CAD build for the part. Positions are in the model's coordinates, mm. Coordinates: 2 decimals unless noted, no trailing zeros. Order: outer loops, then holes, each group sorted by start corner. A loop starts at its lowest first (then second) coordinate and runs counter-clockwise, first axis right, second up. Notation, with made-up numbers: (69, 88) - (128, 88) arc R18 ccw to (128, 100) - close; hole circle Ø9 at (4, 14.25). An arc over 180 degrees is marked (long way). Write each question's results on one line, items separated by ' | '. Start each with the question number.
Q1. Band-saw the part on B-B, the plane x = 27.5. Write the cut outline in (y, z).
Q2. Band-saw the part on D-D, the plane x = -60.5. Write the cut outline in (y, z), then the cut area to 3 significant figures.
Q3. Band-saw the part on A-A, the plane z = 2. Count the separate pieces of the cut face and the enclosed holes in it, then the cut area to 3 significant figures.
Q4. Pin check, flat tip, straight feed: P1, Ø1.5, axis at y = 52, z = 0.5, coming from the +X side. Stop position of the tip, or through.
Q5. Band-saw the part on C-C, the plane y = 20.5. Write the cut outline in (x, z).
Q6. Wall check: probe 1 along Y at (x, z) = (60.5, 1.6); probe 2 along Y at (x, z) = (27.5, 1.4); probe 3 along X at (y, z) = (-56, 0.6). Give the ranges that are in metal, low to high.
Autodesk Inventor part; units mm, degrees
ref_plane "YZ Plane" through (0, 0, 0) normal (1, 0, 0) x (0, 1, 0)
ref_plane "XZ Plane" through (0, 0, 0) normal (0, 1, 0) x (-1, 0, 0)
ref_plane "XY Plane" through (0, 0, 0) normal (0, 0, 1) x (1, 0, 0)
sketch "Sketch1" plane through (0, 0, 0) normal (0, 0, 1) x (1, 0, 0)
  line L0 (-72.5, 65) -> (72.5, 65)
  line L1 (72.5, 65) -> (72.5, -65)
  line L2 (72.5, -65) -> (-72.5, -65)
  line L3 (-72.5, -65) -> (-72.5, 65)
  point P0 (0, 0)
  dimension "d0" = 145
  dimension "d1" = 130
  dimension "d2" = 65
  dimension "d3" = 72.5
extrude "profile" add sketch "Sketch1" along normal blind 2.6568
sketch "Sketch2" plane through (0, 0, 2.6568) normal (0, 0, 1) x (1, 0, 0)
  line L0 (72.5, 65) -> (-72.5, 65)
  line L1 (-72.5, 65) -> (-72.5, -65)
  line L2 (-32.5, 35) -> (-7.5, 35) construction
  line L3 (-32.5, 32.25) -> (-7.5, 32.25)
  line L4 (-7.5, 37.75) -> (-32.5, 37.75)
  arc A0 (-32.5, 37.75) -> (-32.5, 32.25) centre (-32.5, 35) ccw
  arc A1 (-7.5, 32.25) -> (-7.5, 37.75) centre (-7.5, 35) ccw
  point P0 (0, 0)
  point P1 (-20, 35)
  dimension "d6" = 25
  dimension "d7" = 5.5
  dimension "d8" = 30
  dimension "d9" = 40
extrude "x_slots" cut sketch "Sketch2" against normal through all
pattern_linear "Rectangular Pattern1" count 2 spacing 20 along (0, -1, 0) of "x_slots"
sketch "Sketch3" plane through (0, 0, 2.6568) normal (0, 0, 1) x (1, 0, 0)
  line L0 (-72.5, 65) -> (-72.5, -65)
  line L1 (-72.5, -65) -> (72.5, -65)
  circle A0 centre (-60.5, -55) radius 3.57
  circle A1 centre (-60.5, 9.6) radius 2.75
  circle A2 centre (-60.5, 9.6) radius 11.75 construction
  point P0 (0, 0)
  dimension "d15" = 7.14
  dimension "d16" = 5.5
  dimension "d17" = 64.6
  dimension "d18" = 10
  dimension "d19" = 12
  dimension "d21" = 12
extrude "Extrusion3" cut sketch "Sketch3" against normal through all
pattern_linear "Rectangular Pattern2" count 2 spacing 121 along (1, 0, 0) of "Extrusion3"
sketch "Sketch4" plane through (0, 0, 2.6568) normal (0, 0, 1) x (1, 0, 0)
  line L0 (72.5, 65) -> (-72.5, 65)
  line L1 (72.5, -65) -> (72.5, 65)
  circle A0 centre (27.5, 36) radius 11.5
  circle A1 centre (12, 51.5) radius 2
  circle A2 centre (43, 51.5) radius 2
  circle A3 centre (12, 20.5) radius 2
  circle A4 centre (43, 20.5) radius 2
  point P0 (0, 0)
  dimension "d27" = 23
  dimension "d28" = 29
  dimension "d29" = 4
  dimension "d30" = 15.5
  dimension "d31" = 15.5
  dimension "d36" = 45
  dimension "d51" = 31
  dimension "d54" = 31
extrude "nema17_mount" cut sketch "Sketch4" against normal through all
fillet "Fillet1" radius 25 2 edges at (72.5, 65, 1.3284) (-72.5, 65, 1.3284)
sketch "Sketch5" plane through (0, 0, 2.6568) normal (0, 0, 1) x (1, 0, 0)
  line L0 (-72.5, 65) -> (-72.5, -65)
  line L1 (-72.5, -65) -> (72.5, -65)
  circle A0 centre (17.5, 9.5) radius 2.75
  line L2 (47.5, 65) -> (-72.5, 65)
  circle A1 centre (37.5, 9.5) radius 2.75
  point P0 (67.5, -65)
  point P1 (-72.5, 60)
  point P2 (-72.5, -60)
  point P3 (-67.5, -65)
  point P4 (0, 0)
  dimension "d41" = 5.5
  dimension "d42" = 74.5
  dimension "d43" = 90
  dimension "d59" = 20
extrude "idler_holes" cut sketch "Sketch5" against normal through all
fillet "Fillet3" radius 5 2 edges at (-72.5, -65, 1.3284) (72.5, -65, 1.3284)
properties part number "motor_mount_v2" material "Steel, Mild"
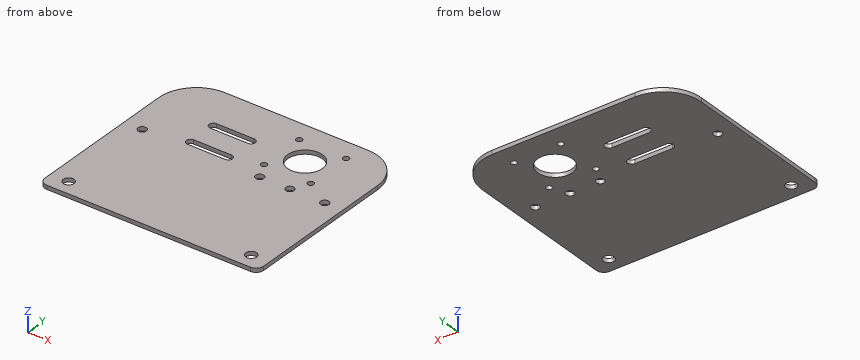
Results below:
1) outline: (-65, 0) - (24.5, 0) - (24.5, 2.66) - (-65, 2.66) - close; (47.5, 0) - (65, 0) - (65, 2.66) - (47.5, 2.66) - close
2) outline: (-65, 0) - (-58.57, 0) - (-58.57, 2.66) - (-65, 2.66) - close; (-51.43, 0) - (6.85, 0) - (6.85, 2.66) - (-51.43, 2.66) - close; (12.35, 0) - (61.35, 0) - (61.35, 2.66) - (12.35, 2.66) - close | area: 302 mm²
3) separate pieces: 1 | enclosed holes: 13 | area: 17,600 mm²
4) P1: stops at x = 69.83
5) outline: (-72.5, 0) - (10, 0) - (10, 2.66) - (-72.5, 2.66) - close; (14, 0) - (41, 0) - (41, 2.66) - (14, 2.66) - close; (45, 0) - (72.5, 0) - (72.5, 2.66) - (45, 2.66) - close
6) probe 1: y = -65 to -58.57, -51.43 to 6.85, 12.35 to 61.35 | probe 2: y = -65 to 24.5, 47.5 to 65 | probe 3: x = -72.5 to -63.93, -57.07 to 57.07, 63.93 to 72.5
